```python
from build123d import *

# Parameters (mm, degrees)
SKETCH1_W            = 180
SKETCH1_H            = 180
BOSS_EXTRUDE1_DEPTH  = 38
SKETCH2_R            = 69
BOSS_EXTRUDE2_DEPTH  = 28
CHAMFER3_SIZE        = 16
CHAMFER3_SIZE2       = 22.850368108
SKETCH3_R            = 36
CUT_EXTRUDE1_DEPTH   = 13
CUT_EXTRUDE2_REACH   = 68
SKETCH4_R            = 31
SKETCH5_R            = 6.5
CUT_EXTRUDE3_DEPTH   = 38
LPATTERN1_COUNT      = 2
LPATTERN1_PITCH      = 140
LPATTERN1_COUNT_DIR2 = 2
LPATTERN1_PITCH_DIR2 = 140
CHAMFER4_SIZE        = 5
CHAMFER5_SIZE        = 1
CHAMFER6_SIZE        = 0.5
FILLET1_R            = 0.3
FILLET2_R            = 3


with BuildPart() as part:
    # Sketch1 → Boss-Extrude1 (new body)
    with BuildSketch(Plane(origin=(0, 0, 0), x_dir=(1, 0, 0), z_dir=(0, 1, 0))):
        Rectangle(SKETCH1_W, SKETCH1_H)
    extrude(amount=BOSS_EXTRUDE1_DEPTH)

    # Sketch2 → Boss-Extrude2 (add)
    with BuildSketch(Plane(origin=(0, 38, 0), x_dir=(1, 0, 0), z_dir=(0, 1, 0))):
        Circle(SKETCH2_R)
    extrude(amount=BOSS_EXTRUDE2_DEPTH)

    # Chamfer3
    chamfer3_edges = [part.edges().sort_by_distance(p)[0] for p in [
        (-69, 66, 0),
    ]]
    chamfer3_side = [part.faces().sort_by_distance(p)[0] for p in [
        (0, 66, 0),
    ]]
    chamfer(chamfer3_edges, length=CHAMFER3_SIZE, length2=CHAMFER3_SIZE2, reference=chamfer3_side[0])

    # Sketch3 → Cut-Extrude1 (cut)
    with BuildSketch(Plane(origin=(0, 66, 0), x_dir=(1, 0, 0), z_dir=(0, 1, 0))):
        Circle(SKETCH3_R)
    extrude(amount=-CUT_EXTRUDE1_DEPTH, mode=Mode.SUBTRACT)

    # Sketch4 → Cut-Extrude2 (cut, up to next)
    with BuildSketch(Plane(origin=(0, 0, 0), x_dir=(-1, 0, 0), z_dir=(0, -1, 0)), mode=Mode.PRIVATE) as cut_extrude2_sk1:
        Circle(SKETCH4_R)
    cut_extrude2_tool1 = extrude(cut_extrude2_sk1.sketch, amount=-CUT_EXTRUDE2_REACH, mode=Mode.PRIVATE) & part.part
    add(cut_extrude2_tool1.solids().sort_by_distance((0, 0, 0))[0], mode=Mode.SUBTRACT)

    # Sketch5 → Cut-Extrude3 (cut)
    with BuildSketch(Plane(origin=(0, 38, 0), x_dir=(1, 0, 0), z_dir=(0, 1, 0))):
        with Locations((-70, 70)):
            Circle(SKETCH5_R)
    cut_extrude3 = extrude(amount=-CUT_EXTRUDE3_DEPTH, mode=Mode.SUBTRACT)

    # LPattern1: Cut-Extrude3 2 × 2
    with Locations(*[(i * LPATTERN1_PITCH, 0, j * LPATTERN1_PITCH_DIR2) for i in range(LPATTERN1_COUNT) for j in range(LPATTERN1_COUNT_DIR2) if (i, j) != (0, 0)]):
        add(cut_extrude3, mode=Mode.SUBTRACT)

    # Chamfer4
    chamfer4_edges = [part.edges().sort_by_distance(p)[0] for p in [
        (-90, 19, -90),
        (90, 19, -90),
        (90, 19, 90),
        (-90, 19, 90),
    ]]
    chamfer(chamfer4_edges, length=CHAMFER4_SIZE)

    # Chamfer5
    chamfer5_edges = [part.edges().sort_by_distance(p)[0] for p in [
        (31, 53, 0),
        (31, 0, 0),
    ]]
    chamfer(chamfer5_edges, length=CHAMFER5_SIZE)

    # Chamfer6
    chamfer6_edges = [part.edges().sort_by_distance(p)[0] for p in [
        (-36, 66, 0),
    ]]
    chamfer(chamfer6_edges, length=CHAMFER6_SIZE)

    # Fillet1
    fillet1_edges = [part.edges().sort_by_distance(p)[0] for p in [
        (-36, 53, 0),
    ]]
    fillet(fillet1_edges, radius=FILLET1_R)

    # Fillet2
    fillet2_edges = [part.edges().sort_by_distance(p)[0] for p in [
        (-69, 38, 0),
    ]]
    fillet(fillet2_edges, radius=FILLET2_R)


solid = part.part
```
The model under review builds one solid part; all positions refer to its coordinate system, in mm. A direction names the side the tool comes from. Round coordinates to 2 decimals unless told otherwise and drop trailing zeros. Order: outer loops, then holes, each group sorted by start corner. A loop starts at its lowest first (then second) coordinate and runs counter-clockwise, first axis right, second up.
Item 1: For pin 1 (5 mm diameter, centred on y = 46, z = 30.5, fed in from -X); pin 2 (10.5 mm diameter, centred on x = -70, z = 70, fed in from +Y); pin 3 (15 mm diameter, centred on x = 70, z = -70, fed in from +Y); pin 4 (1 mm diameter, centred on x = 40, z = -41, fed in from +Y), all flat-tipped, find the tip position at first contact; note any pin that passes through.
Working result:
pin 1: stops at x = -61.96
pin 2: passes through
pin 3: stops at y = 38
pin 4: stops at y = 60.6
Item 2: Add section B-B, the plane y = 27. State the section outline as (x, z) points.
Working result:
outline: (-90, -85) - (-85, -90) - (85, -90) - (90, -85) - (90, 85) - (85, 90) - (-85, 90) - (-90, 85) - close; hole circle Ø13 at (-70, -70); hole circle Ø13 at (-70, 70); hole circle Ø62 at (0, 0); hole circle Ø13 at (70, -70); hole circle Ø13 at (70, 70)
Item 3: To check wall thickness, follow probe 1 along X at (y, z) = (15, 70); probe 2 along X at (y, z) = (22.5, 0). State the ranges of each line that lie inside material, in increasing order.
Working result:
probe 1: x = -90 to -76.5, -63.5 to 63.5, 76.5 to 90
probe 2: x = -90 to -31, 31 to 90
Item 4: Add section A-A, the plane x = 0. State the section outline as (y, z) points.
Working result:
outline: (0, -90) - (38, -90) - (38, -72) arc R3 cw to (41, -69) - (43.15, -69) - (66, -53) - (66, -36.5) - (65.5, -36) - (53.3, -36) arc R0.3 cw to (53, -35.7) - (53, -32) - (52, -31) - (1, -31) - (0, -32) - close; (0, 32) - (1, 31) - (52, 31) - (53, 32) - (53, 35.7) arc R0.3 cw to (53.3, 36) - (65.5, 36) - (66, 36.5) - (66, 53) - (43.15, 69) - (41, 69) arc R3 cw to (38, 72) - (38, 90) - (0, 90) - close
Item 5: Draft analysis for pull direction Z (two halves, no side actions). For faces 3 (the flat face through (-87, 19, 88)), 4 (the cylindrical face through (72.999, 19.266, 75.767)), 5 (the flat face through (-90, 19, 1)), state which applies: released by +Z, released by -Z, zero draft, split by the parting line, or undercut.
Working result:
face 3: released by +Z
face 4: undercut
face 5: zero draft
Item 6: Machinability: for faces 1 (the flat face through (-61, 38, -41)), 2 (the cylindrical face through (-67.001, 19.266, -64.233)), which of the approach directions +Z, -Z, +X, -X, +Y, -Y give a long, thin tool a straight path to every point of the face, cutting with its end or side? Answer none if there is none.
Working result:
face 1: +Y
face 2: +Y, -Y
Item 7: Add section C-C, the plane z = 0. State the section outline as (x, y) points.
Working result:
outline: (-90, 0) - (-32, 0) - (-31, 1) - (-31, 52) - (-32, 53) - (-35.7, 53) arc R0.3 cw to (-36, 53.3) - (-36, 65.5) - (-36.5, 66) - (-53, 66) - (-69, 43.15) - (-69, 41) arc R3 cw to (-72, 38) - (-90, 38) - close; (31, 1) - (32, 0) - (90, 0) - (90, 38) - (72, 38) arc R3 cw to (69, 41) - (69, 43.15) - (53, 66) - (36.5, 66) - (36, 65.5) - (36, 53.3) arc R0.3 cw to (35.7, 53) - (32, 53) - (31, 52) - close
